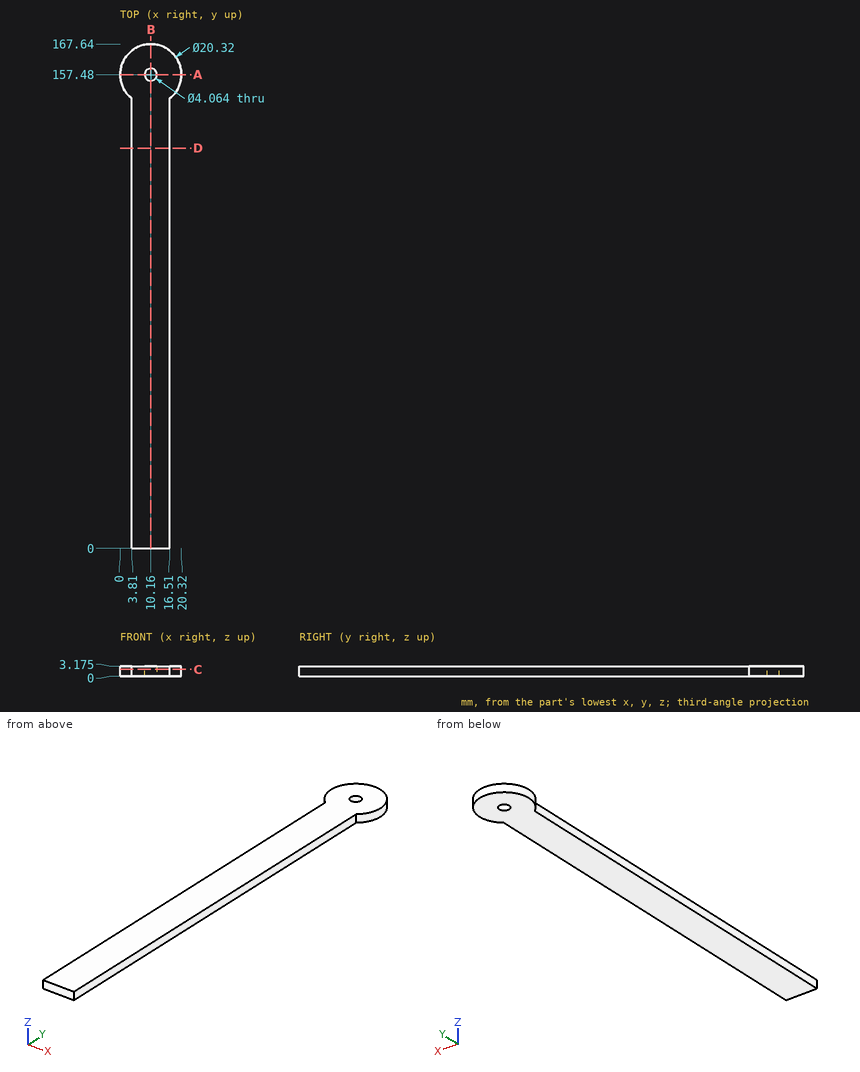
Study the drawing (mm; zero at the part's minimum x, y, z) and answer. Give positions to 0.01 mm unless a question says otherwise; leave off trailing zeros. Order: outer loops, then holes, each group sorted by start corner. A loop starts at its lowest first (then second) coordinate and runs counter-clockwise, first axis right, second up. Notation, with made-up numbers: (-26.5, 46) -> (2.5, 46) arc R15 cw to (2.5, 59) -> close; hole circle Ø11 at (7.25, 30.5). An arc over 180 degrees is marked (long way). Write item = value, one per line.
1. Given pin 1 (1 mm diameter, centred on y = 60, z = 2, fed in from -X); pin 2 (2 mm diameter, centred on x = 2.5, y = 57, fed in from -Z), each flat-ended and moving along its own axis, determine where each tip first touches the part or whether it passes through.
Numbers:
pin_1 = 3.81
pin_2 = through
2. A cutting plane is placed at C-C, the plane z = 2.2. Write down the section's boundary in (x, y), and give its area (3 significant figures).
Numbers:
outline = (3.81, 0) -> (16.51, 0) -> (16.51, 149.55) arc R10.16 ccw (long way) to (3.81, 149.55) -> close; hole circle Ø4.06 at (10.16, 157.48)
area = 2,190 mm²
3. A cutting plane is placed at D-D, the plane y = 133. Write down the section's boundary in (x, z) (3 decimals).
Numbers:
outline = (3.81, 0) -> (16.51, 0) -> (16.51, 3.175) -> (3.81, 3.175) -> close
4. A cutting plane is placed at A-A, the plane y = 157.48. Write down the section's boundary in (x, z) (3 decimals), and give its area (3 significant figures).
Numbers:
outline = (0, 0) -> (8.128, 0) -> (8.128, 3.175) -> (0, 3.175) -> close; (12.192, 0) -> (20.32, 0) -> (20.32, 3.175) -> (12.192, 3.175) -> close
area = 51.6 mm²
5. Straight lines are drawn through the part: line 1 along Y through (x, z) = (10.16, 1.7); line 2 along X through (y, z) = (157.48, 2.3); line 3 along X through (y, z) = (40, 2.35). For each, find the intervals that lie inside material, in ascending order.
Numbers:
line_1 = 0 to 155.45, 159.51 to 167.64
line_2 = 0 to 8.13, 12.19 to 20.32
line_3 = 3.81 to 16.51
6. A cutting plane is placed at B-B, the plane x = 10.16. Write down the section's boundary in (y, z) (3 decimals), and give its area (3 significant figures).
Numbers:
outline = (0, 0) -> (155.448, 0) -> (155.448, 3.175) -> (0, 3.175) -> close; (159.512, 0) -> (167.64, 0) -> (167.64, 3.175) -> (159.512, 3.175) -> close
area = 519 mm²
